Could you check a few things on this drawing? It's one solid part, dimensions in mm from its lowest x, y, z. A direction names the side the tool comes from. Round coordinates to 2 decimals unless told otherwise and drop trailing zeros. Write each loop counter-clockwise with the first axis right and the second up, starting at its lowest first coordinate (ties: lowest second). Pieces come first, ordered by that corner, then holes. Notation, with made-up numbers: (60.5, -1) -> (95.5, -1) arc R3 ccw to (95.5, 4) -> close; hole circle Ø3 at (45.5, -15). An arc over 180 degrees is marked (long way). Answer as CSV lines item,"result".
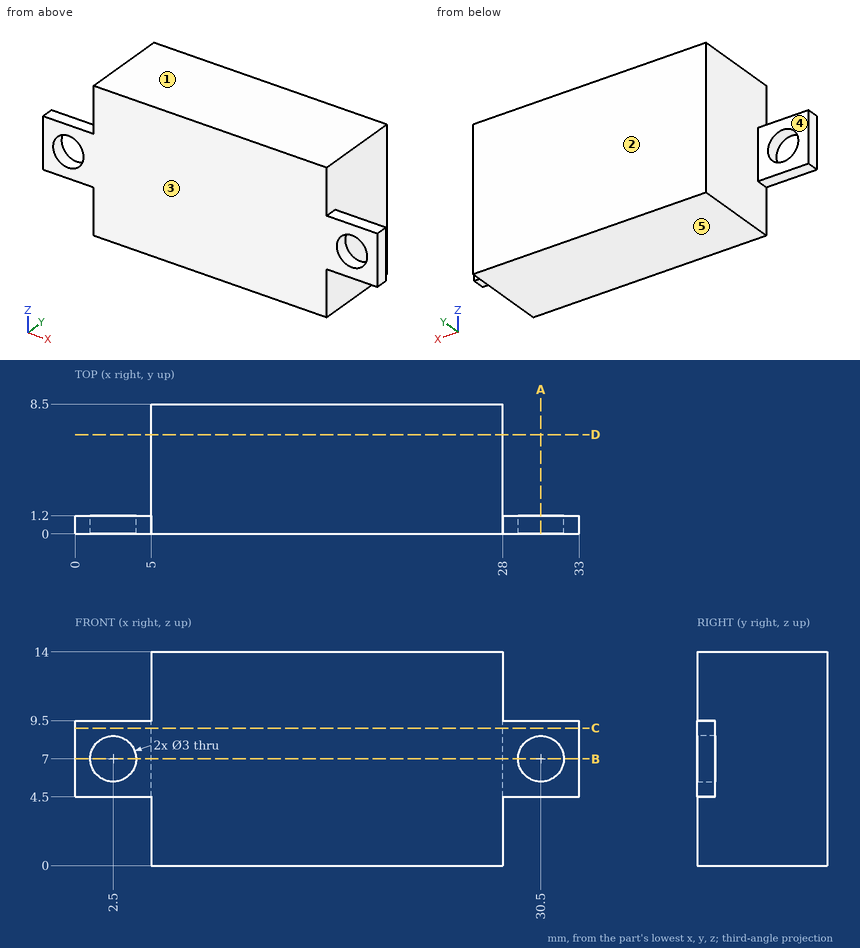
1. Suppose I cut it at B-B on z = 7. Please give me the cut outline in (x, y).
Numbers:
outline,"(0, 0) -> (1, 0) -> (1, 1.2) -> (0, 1.2) -> close; (4, 0) -> (29, 0) -> (29, 1.2) -> (28, 1.2) -> (28, 8.5) -> (5, 8.5) -> (5, 1.2) -> (4, 1.2) -> close; (32, 0) -> (33, 0) -> (33, 1.2) -> (32, 1.2) -> close"
2. On a 3-axis mill with a long thin cutter (end or side, diameter ignored), from which of +Z, -Z, +X, -X, +Y, -Y can I reach the whole of each face in a straight line? I mean the marked faces 4 and 5. Say none if no direction works.
Numbers:
face 4,"+Z, -Z, -X, +Y"
face 5,"-Z, +X, -X, +Y, -Y"
3. Suppose I cut it at A-A on x = 30.5. Please give me the cut outline in (y, z), and give its area (3 significant figures).
Numbers:
outline,"(0, 4.5) -> (1.2, 4.5) -> (1.2, 5.5) -> (0, 5.5) -> close; (0, 8.5) -> (1.2, 8.5) -> (1.2, 9.5) -> (0, 9.5) -> close"
area,"2.40 mm^2"
4. Suppose I cut it at C-C on z = 9. Please give me the cut outline in (x, y).
Numbers:
outline,"(0, 0) -> (33, 0) -> (33, 1.2) -> (28, 1.2) -> (28, 8.5) -> (5, 8.5) -> (5, 1.2) -> (0, 1.2) -> close"
5. For pin 1 Ø4 at (x, z) = (2.5, 6) entering from +Y; pin 2 Ø2.5 at (y, z) = (3, 6.5) entering from -X; pin 3 Ø1.3 at (x, y) = (2.5, 1) entering from +Z, each with a flat end and sliding along its axis, tell me the tip position at first contact or that it passes through.
Numbers:
pin 1,"stops at y = 1.2"
pin 2,"stops at x = 5"
pin 3,"stops at z = 9.5"
6. If we mould it in two halves opening along Y, with no side actions, what happens to the marked faces 1, 2 and 3? For each: released by +Y, released by -Y, zero draft, split by the parting line, or undercut.
Numbers:
face 1,"zero draft"
face 2,"released by +Y"
face 3,"released by -Y"
7. If I drill on line 1 (X direction, y = 0.25, z = 7); line 2 (X direction, y = 5, z = 5); line 3 (Y direction, x = 32, z = 5.25), over which ranges is the centre line in solid material (lowest first)?
Numbers:
line 1,"x = 0 to 1, 4 to 29, 32 to 33"
line 2,"x = 5 to 28"
line 3,"y = 0 to 1.2"
8. Suppose I cut it at D-D on y = 6.5. Please give me the cut outline in (x, z).
Numbers:
outline,"(5, 0) -> (28, 0) -> (28, 14) -> (5, 14) -> close"
